```python
from build123d import *

# Parameters (mm, degrees)
F1_DEPTH = 43
F2_W     = 39
F2_H     = 7
F4_W     = 39
F4_H     = 7
F6_W     = 39
F6_H     = 7
F7_ANGLE = -20.8


with BuildPart() as f1:
    # F0 (on Top) → F1 (new body)
    with BuildSketch(Plane.XY):
        with BuildLine():
            Line((-12.5, -22.5), (12.5, -22.5))
            ThreePointArc((12.5, -22.5), (19.571068, -19.571068), (22.5, -12.5))
            Line((22.5, -12.5), (22.5, 12.5))
            ThreePointArc((22.5, 12.5), (19.571068, 19.571068), (12.5, 22.5))
            Line((12.5, 22.5), (-12.5, 22.5))
            ThreePointArc((-12.5, 22.5), (-19.571068, 19.571068), (-22.5, 12.5))
            Line((-22.5, 12.5), (-22.5, -12.5))
            ThreePointArc((-22.5, -12.5), (-19.571068, -19.571068), (-12.5, -22.5))
        make_face()
    extrude(amount=F1_DEPTH)

    # F2 (on face) → F5 section 0
    with BuildSketch(Plane.XY.offset(43)):
        Rectangle(F2_W, F2_H)
    # F4 (on offset) → F5 section 1
    with BuildSketch(Plane.XY.offset(5)):
        with Locations((0, -10.5)):
            Rectangle(F4_W, F4_H)
    loft(mode=Mode.SUBTRACT)

    # F6 (on face) → F7 (revolve)
    with BuildSketch(Plane.XY.offset(5)):
        with Locations((0, -10.5)):
            Rectangle(F6_W, F6_H)
    revolve(axis=Axis((0, -7, 5), (1, 0, 0)), revolution_arc=F7_ANGLE)


solid = f1.part
```
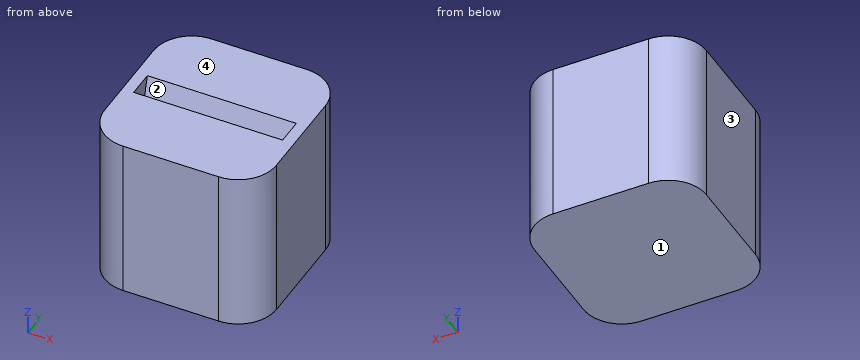
Verification items for the finished model (mm, model axes). Face numbers are marked on the shaded views. Coordinates: 2 decimals unless noted, no trailing zeros. Loops run counter-clockwise (first coordinate to the right, second up) from the corner with the lowest first, then second, coordinate; pieces in that order, holes last. Notation, with made-up numbers: (19, 35) - (76, 35) arc R11 ccw to (76, 50) - close; hole circle Ø2 at (-10, 52.25). An arc over 180 degrees is marked (long way). Answer as a JSON object with one key per item and string values.
(1) Cross-section at B-B, the plane z = 3. Record the boundary of the cut face in (x, y), then the cut area to 3 significant figures.
Response:
{"outline": "(-22.5, -12.5) arc R10 ccw to (-12.5, -22.5) - (12.5, -22.5) arc R10 ccw to (22.5, -12.5) - (22.5, 12.5) arc R10 ccw to (12.5, 22.5) - (-12.5, 22.5) arc R10 ccw to (-22.5, 12.5) - close", "area": "1,940 mm²"}
(2) Cross-section at C-C, the plane y = -16. Record the boundary of the cut face in (x, z), then the cut area to 3 significant figures.
Response:
{"outline": "(-21.87, 0) - (21.87, 0) - (21.87, 43) - (-21.87, 43) - close", "area": "1,880 mm²"}
(3) Mould release check, pull along Z, two halves, no side actions. Record for the marked faces 1, 2, 3 and 4: pulls with the +Z half, pulls with the -Z half, needs draft (parallel to the pull), parting line crosses it, or undercut.
Response:
{"face 1": "pulls with the -Z half", "face 2": "undercut", "face 3": "needs draft", "face 4": "pulls with the +Z half"}
(4) Scan lines: line 1 along X through (y, z) = (-6.5, 30); line 2 along X through (y, z) = (-13, 17); line 3 along Y through (x, z) = (11, 36.5). Record each from-to range of solid material in increasing order.
Response:
{"line 1": "x = -22.5 to -19.5, 19.5 to 22.5", "line 2": "x = -22.49 to 22.49", "line 3": "y = -22.5 to -5.3, 1.7 to 22.5"}
(5) Cross-section at A-A, the plane x = 3.5. Record the boundary of the cut face in (y, z).
Response:
{"outline": "(-22.5, 0) - (22.5, 0) - (22.5, 43) - (3.5, 43) - (-7, 5) - (-13.34, 7.41) - (-3.5, 43) - (-22.5, 43) - close"}
